```python
from build123d import *

# Parameters (mm, degrees)
SKETCH_1_W          = 15
SKETCH_1_H          = 120
EXTRUDE_1_DEPTH     = 6
SKETCH_2_R          = 1.65
CUT_EXTRUDE_1_DEPTH = 61.763887302
SKETCH_3_W          = 5.8
SKETCH_3_H          = 15.8
CUT_EXTRUDE_2_DEPTH = 3.1
CUT_EXTRUDE_3_DEPTH = 3.1
SKETCH_5_R          = 2.9
CUT_EXTRUDE_4_DEPTH = 3.2
SKETCH_6_W          = 7.5
SKETCH_6_H          = 10
EXTRUDE_2_DEPTH     = 4
SKETCH_7_W          = 13.5
SKETCH_7_H          = 16
EXTRUDE_3_DEPTH     = 2


with BuildPart() as part:
    # 草图1 → 凸台-拉伸1 (new body)
    with BuildSketch(Plane.XY):
        Rectangle(SKETCH_1_W, SKETCH_1_H)
    extrude(amount=EXTRUDE_1_DEPTH)

    # 草图2 → 切除-拉伸1 (cut, through all)
    with BuildSketch(Plane.XY.offset(6)):
        with Locations((0, 50)):
            Circle(SKETCH_2_R)
        with Locations(Location((0, -50, 0), (0, 0, 180))):
            Circle(SKETCH_2_R)
    extrude(amount=-CUT_EXTRUDE_1_DEPTH, mode=Mode.SUBTRACT)

    # 草图3 → 切除-拉伸2 (cut)
    with BuildSketch(Plane(origin=(0, 0, 0), x_dir=(-1, 0, 0), z_dir=(0, 0, -1))):
        with Locations((0, -5.44)):
            Rectangle(SKETCH_3_W, SKETCH_3_H)
    extrude(amount=-CUT_EXTRUDE_2_DEPTH, mode=Mode.SUBTRACT)

    # 草图4 → 切除-拉伸3 (cut)
    with BuildSketch(Plane(origin=(0, 0, 0), x_dir=(-1, 0, 0), z_dir=(0, 0, -1))):
        Polygon((-2.9, 2.46), (0, 5.36), (2.9, 2.46), align=None)
    extrude(amount=-CUT_EXTRUDE_3_DEPTH, mode=Mode.SUBTRACT)

    # 草图5 → 切除-拉伸4 (cut)
    with BuildSketch(Plane.XY.offset(6)):
        with Locations((0, 50)):
            Circle(SKETCH_5_R)
        with Locations((0, -50)):
            Circle(SKETCH_5_R)
    extrude(amount=-CUT_EXTRUDE_4_DEPTH, mode=Mode.SUBTRACT)

    # 草图6 → 凸台-拉伸2 (add)
    with BuildSketch(Plane.XY.offset(6)):
        with Locations((-3.75, -15)):
            Rectangle(SKETCH_6_W, SKETCH_6_H)
        with Locations((-3.75, 25)):
            Rectangle(SKETCH_6_W, SKETCH_6_H)
    extrude(amount=EXTRUDE_2_DEPTH)

    # 草图7 → 凸台-拉伸3 (add)
    with BuildSketch(Plane.XY.offset(10)):
        with Locations((-3.75, 25)):
            Rectangle(SKETCH_7_W, SKETCH_7_H)
        with Locations((-3.75, -15)):
            Rectangle(SKETCH_7_W, SKETCH_7_H)
    extrude(amount=EXTRUDE_3_DEPTH)


solid = part.part
```
Build history of the part. All positions in model axes, mm. A direction names the side the tool comes from. Round coordinates to 2 decimals unless told otherwise and drop trailing zeros. Loops run counter-clockwise (first coordinate to the right, second up) from the corner with the lowest first, then second, coordinate; pieces in that order, holes last.
Item 1: Saw through at B-B (y = -50). List the corners of the cut face in (x, z), then the cut area to 3 significant figures.
Item 2: Drill centre lines: line 1 along Y through (x, z) = (0, 1.55); line 2 along Y through (x, z) = (0, 4.2); line 3 along X through (y, z) = (-6, 0.5). Where is each one in solid material? Low to high.
Item 3: Saw through at A-A (z = 7). List the corners of the cut face in (x, y).
Item 4: Saw through at D-D (z = 1.75). List the corners of the cut face in (x, y).
Item 5: Which spindle directions (+Z, -Z, +X, -X, +Y, -Y) get a long thin tool onto all of the face, cutting with end or side? Do faces 4 (the face through (-8, -15, 10)), 5 (the face through (3, 25, 11)), 6 (the face through (-4, 20, 8)), 7 (the face through (-4, 17, 11)). Say none if no direction does.
Item 6: Saw through at C-C (x = -5). List the corners of the cut face in (y, z), then the cut area to 3 significant figures.
Item 7: Pin check, flat tips, straight feed: P1, Ø5.5, axis at x = 0, y = 50, coming from the +Z side; P2, Ø7.5, axis at x = -2, y = -4.5, coming from the +Z side; P3, Ø4.5, axis at x = -0.5, y = 50.5, coming from the +Z side; P4, Ø1.2, axis at x = -2, z = 8, coming from the +Y side. Stop position of each tip, or through.
Item 8: Two-plate mould, pull along Z, no slides. Class faces 1 (the face through (-2.9, -6, 2)), 2 (the face through (2, 50, 2.8)), 3 (the face through (0, -15, 8)): released by +Z, released by -Z, zero draft, split by the parting line, or undercut.
Worked answers:
1. outline: (-7.5, 0) - (-1.65, 0) - (-1.65, 2.8) - (-2.9, 2.8) - (-2.9, 6) - (-7.5, 6) - close; (1.65, 0) - (7.5, 0) - (7.5, 6) - (2.9, 6) - (2.9, 2.8) - (1.65, 2.8) - close
1. area: 62.2 mm2
2. line 1: y = -60 to -51.65, -48.35 to -13.34, 5.36 to 48.35, 51.65 to 60
2. line 2: y = -60 to -52.9, -47.1 to 47.1, 52.9 to 60
2. line 3: x = -7.5 to -2.9, 2.9 to 7.5
3. outline: (-7.5, -20) - (0, -20) - (0, -10) - (-7.5, -10) - close; (-7.5, 20) - (0, 20) - (0, 30) - (-7.5, 30) - close
4. outline: (-7.5, -60) - (7.5, -60) - (7.5, 60) - (-7.5, 60) - close; hole (-2.9, -13.34) - (2.9, -13.34) - (2.9, 2.46) - (0, 5.36) - (-2.9, 2.46) - close; hole circle Ø3.3 at (0, -50); hole circle Ø3.3 at (0, 50)
5. face 4: none
5. face 5: +Z, +X, +Y, -Y
5. face 6: +X, -X
5. face 7: +Z, +X, -X
6. outline: (-60, 0) - (60, 0) - (60, 6) - (30, 6) - (30, 10) - (33, 10) - (33, 12) - (17, 12) - (17, 10) - (20, 10) - (20, 6) - (-10, 6) - (-10, 10) - (-7, 10) - (-7, 12) - (-23, 12) - (-23, 10) - (-20, 10) - (-20, 6) - (-60, 6) - close
6. area: 864 mm2
7. P1: stops at z = 2.8
7. P2: stops at z = 12
7. P3: stops at z = 6
7. P4: stops at y = 30
8. face 1: zero draft
8. face 2: released by +Z
8. face 3: undercut
